Geometry check sheet. Reference: the model listing, model coordinates, mm. Face numbers are marked on the shaded views. A direction names the side the tool comes from. Coordinates: 2 decimals unless noted, no trailing zeros. Write each loop counter-clockwise with the first axis right and the second up, starting at its lowest first coordinate (ties: lowest second). Pieces come first, ordered by that corner, then holes. Notation, with made-up numbers: M 31.5,31.25 L 60.5,31.25 A18 cw 60.5,42.25 Z; hole C 28.25,-31.75 d9. An arc over 180 degrees is marked long. Put each result on its own line as item: value. Start each with the question number.
1) Cross-section at B-B on x = 0. Record the cut outline in (y, z).
2) Cross-section at C-C on y = 4. Count the separate pieces of the cut face and the enclosed holes in it, plus the area to 3 significant figures.
3) Set-up check for the marked faces 4, 5 and 6: record each of +Z, -Z, +X, -X, +Y, -Y from which the full face is reachable in a straight line by a thin tool's end or side.
4) Gauge pin test, flat ends, axial feed: pin 1 (1.6 mm diameter, centred on x = -7.5, z = 26.4, fed in from +Y); pin 2 (7 mm diameter, centred on x = 18, y = -4.5, fed in from -Z); pin 3 (7 mm diameter, centred on x = 16.5, y = -3, fed in from +Z). Record the tip position at first contact, or that the pin passes through.
5) Mould release check, pull along Z, two halves, no side actions. Record for the marked faces 1, 2 and 3: released by +Z, released by -Z, zero draft, split by the parting line, or undercut.
6) Cross-section at A-A on z = -5. Record the cut outline in (x, y), plus the area to 4 significant figures.
7) Scan lines: line 1 along X through (y, z) = (5, 29); line 2 along X through (y, z) = (-1.75, -5.5); line 3 along Z through (x, y) = (-22.5, -1.25). Record each from-to range of solid material in increasing order.
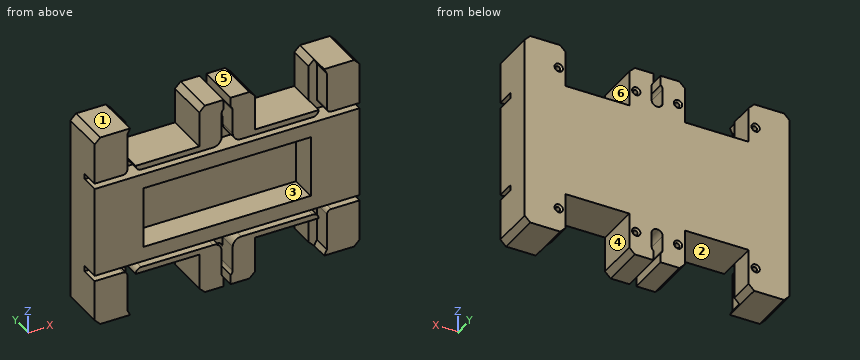
from build123d import *
from build123d.topology import SkipClean

# Parameters (mm, degrees)
SKETCH1_W            = 95
SKETCH1_H            = 70
BOSS_EXTRUDE1_DEPTH  = 7.85
CUT_EXTRUDE1_DEPTH   = 62.055220907
CHAMFER1_SIZE        = 2
CUT_EXTRUDE2_DEPTH   = 6.5
CUT_EXTRUDE3_DEPTH   = 60.715073474
MIRROR3_COPY_1_DEPTH = 6.5
SKETCH7_W            = 60
SKETCH7_H            = 22
CUT_EXTRUDE4_DEPTH   = 9.5


# Read off the part's stored shape, not the designer's step: CSK for M2 Flat Head Machine Screw1
with BuildPart() as part:
    # Sketch1 → Boss-Extrude1 (new, symmetric)
    with BuildSketch(Plane(origin=(0, 0, 0), x_dir=(1, 0, 0), z_dir=(0, 1, 0))):
        Rectangle(SKETCH1_W, SKETCH1_H)
    extrude(amount=BOSS_EXTRUDE1_DEPTH, both=True)

    # Sketch2 → Cut-Extrude1 (cut, through all)
    with BuildSketch(Plane(origin=(0, 7.85, 0), x_dir=(1, 0, 0), z_dir=(0, 1, 0))):
        Polygon((-32.8, -32.5), (-32.8, -20.3), (-10, -20.3), (-10, -32.5), (-10, -35), (-32.8, -35), align=None)
        Polygon((10, -32.5), (10, -20.3), (32.8, -20.3), (32.8, -32.5), (32.8, -35), (10, -35), align=None)
    cut_extrude1 = extrude(amount=-CUT_EXTRUDE1_DEPTH, mode=Mode.SUBTRACT)

    # CSK for M2 Flat Head Machine Screw1 outl → CSK for M2 Flat Head Machine Screw1 (revolve, cut)
    with BuildSketch(Plane(origin=(35.3, 0, 26.4), x_dir=(1, 0, 0), z_dir=(0, 0, 1))):
        Polygon((0, 7.85), (0, -0.672748739), (0.87, -0.15), (0.87, 7.22), (1.5, 7.85), align=None)
    csk_for_m2_flat_head_machine_screw1 = revolve(axis=Axis((35.3, 0, 26.4), (0, 1, 0)), mode=Mode.SUBTRACT)

    # CSK for M2 Flat Head Machine Screw1 2 ou → CSK for M2 Flat Head Machine Screw1 2 (revolve, cut)
    with BuildSketch(Plane(origin=(7.5, 0, 26.4), x_dir=(1, 0, 0), z_dir=(0, 0, 1))):
        Polygon((0, 7.85), (0, -0.672748739), (0.87, -0.15), (0.87, 7.22), (1.5, 7.85), align=None)
    csk_for_m2_flat_head_machine_screw1_2 = revolve(axis=Axis((7.5, 0, 26.4), (0, 1, 0)), mode=Mode.SUBTRACT)

    # CSK for M2 Flat Head Machine Screw1 3 ou → CSK for M2 Flat Head Machine Screw1 3 (revolve, cut)
    with BuildSketch(Plane(origin=(-7.5, 0, 26.4), x_dir=(1, 0, 0), z_dir=(0, 0, 1))):
        Polygon((0, 7.85), (0, -0.672748739), (0.87, -0.15), (0.87, 7.22), (1.5, 7.85), align=None)
    csk_for_m2_flat_head_machine_screw1_3 = revolve(axis=Axis((-7.5, 0, 26.4), (0, 1, 0)), mode=Mode.SUBTRACT)

    # CSK for M2 Flat Head Machine Screw1 4 ou → CSK for M2 Flat Head Machine Screw1 4 (revolve, cut)
    with BuildSketch(Plane(origin=(-35.3, 0, 26.4), x_dir=(1, 0, 0), z_dir=(0, 0, 1))):
        Polygon((0, 7.85), (0, -0.672748739), (0.87, -0.15), (0.87, 7.22), (1.5, 7.85), align=None)
    csk_for_m2_flat_head_machine_screw1_4 = revolve(axis=Axis((-35.3, 0, 26.4), (0, 1, 0)), mode=Mode.SUBTRACT)

    # Mirror1: Cut-Extrude1, CSK for M2 Flat Head Machine Screw1, CSK for M2 Flat Head Machine Screw1 2, CSK for M2 Flat Head Machine Screw1 3, CSK for M2 Flat Head Machine Screw1 4 across plane
    add(cut_extrude1.mirror(Plane.XY), mode=Mode.SUBTRACT)
    add(csk_for_m2_flat_head_machine_screw1.mirror(Plane.XY), mode=Mode.SUBTRACT)
    add(csk_for_m2_flat_head_machine_screw1_2.mirror(Plane.XY), mode=Mode.SUBTRACT)
    add(csk_for_m2_flat_head_machine_screw1_3.mirror(Plane.XY), mode=Mode.SUBTRACT)
    add(csk_for_m2_flat_head_machine_screw1_4.mirror(Plane.XY), mode=Mode.SUBTRACT)

    # Chamfer1
    chamfer1_edges = [part.edges().sort_by_distance(p)[0] for p in [
        (-32.8, 0, 35),
        (-10, 0, 35),
        (10, 0, 35),
        (32.8, 0, 35),
        (47.5, 0, 35),
        (-47.5, 0, 35),
        (-47.5, 0, -35),
        (47.5, 0, -35),
        (-32.8, 0, -35),
        (-10, 0, -35),
        (10, 0, -35),
        (32.8, 0, -35),
    ]]
    chamfer(chamfer1_edges, length=CHAMFER1_SIZE)

    # Sketch5 → Cut-Extrude2 (cut)
    with BuildSketch(Plane.XZ.offset(7.85)):
        with BuildLine():
            Line((47.5, 16.3), (-2, 16.3))
            Line((-2, 16.3), (-2, 30))
            ThreePointArc((-2, 30), (0, 32), (2, 30))
            Line((2, 30), (2, 21.3))
            ThreePointArc((2, 21.3), (2.878679656, 19.178679656), (5, 18.3))
            Line((5, 18.3), (30.8, 18.3))
            ThreePointArc((30.8, 18.3), (32.214213562, 18.885786438), (32.8, 20.3))
            Line((32.8, 20.3), (32.8, 33))
            Line((32.8, 33), (34.8, 35))
            Line((34.8, 35), (35.8, 33))
            Line((35.8, 33), (35.8, 19.8))
            ThreePointArc((35.8, 19.8), (36.239339828, 18.739339828), (37.3, 18.3))
            Line((37.3, 18.3), (47.5, 18.3))
            Line((47.5, 18.3), (47.5, 16.3))
        make_face()
    cut_extrude2 = extrude(amount=-CUT_EXTRUDE2_DEPTH, mode=Mode.SUBTRACT)

    # Sketch6 → Cut-Extrude3 (cut, symmetric)
    with SkipClean():  # the faces are left unmerged after this step: merging them gives an invalid solid
        with BuildSketch(Plane.XZ.offset(1.35)):
            with BuildLine():
                Line((2, 25), (2, 30))
                ThreePointArc((2, 30), (1.802775638, 30.866025404), (1.25, 31.5612495))
                Line((1.25, 31.5612495), (1.25, 35))
                Line((1.25, 35), (-1.25, 35))
                Line((-1.25, 35), (-1.25, 31.5612495))
                ThreePointArc((-1.25, 31.5612495), (-1.802775638, 30.866025404), (-2, 30))
                Line((-2, 30), (-2, 25))
                ThreePointArc((-2, 25), (0, 23), (2, 25))
            make_face()
        cut_extrude3 = extrude(amount=CUT_EXTRUDE3_DEPTH, both=True, mode=Mode.SUBTRACT)
    add(part.part.scale(1), mode=Mode.REPLACE)  # the faces are merged on a copy

    # Mirror2: Cut-Extrude2 across plane
    add(cut_extrude2.mirror(Plane(origin=(0, 0, 0), x_dir=(0, 0, 1), z_dir=(1, 0, 0))), mode=Mode.SUBTRACT)

    # Mirror3: Cut-Extrude2, Cut-Extrude3 across plane
    add(cut_extrude2.mirror(Plane.XY), mode=Mode.SUBTRACT)
    add(cut_extrude3.mirror(Plane.XY), mode=Mode.SUBTRACT)

    # Mirror3 copy 1 sketch → Mirror3 copy 1 (cut)
    with BuildSketch(Plane(origin=(0, -7.85, 0), x_dir=(-1, 0, 0), z_dir=(0, -1, 0))):
        with BuildLine():
            Line((47.5, 16.3), (-2, 16.3))
            Line((-2, 16.3), (-2, 30))
            ThreePointArc((-2, 30), (0, 32), (2, 30))
            Line((2, 30), (2, 21.3))
            ThreePointArc((2, 21.3), (2.878679656, 19.178679656), (5, 18.3))
            Line((5, 18.3), (30.8, 18.3))
            ThreePointArc((30.8, 18.3), (32.214213562, 18.885786438), (32.8, 20.3))
            Line((32.8, 20.3), (32.8, 33))
            Line((32.8, 33), (34.8, 35))
            Line((34.8, 35), (35.8, 33))
            Line((35.8, 33), (35.8, 19.8))
            ThreePointArc((35.8, 19.8), (36.239339828, 18.739339828), (37.3, 18.3))
            Line((37.3, 18.3), (47.5, 18.3))
            Line((47.5, 18.3), (47.5, 16.3))
        make_face()
    extrude(amount=-MIRROR3_COPY_1_DEPTH, mode=Mode.SUBTRACT)

    # Sketch7 → Cut-Extrude4 (cut)
    with BuildSketch(Plane.XZ.offset(7.85)):
        Rectangle(SKETCH7_W, SKETCH7_H)
    extrude(amount=-CUT_EXTRUDE4_DEPTH, mode=Mode.SUBTRACT)


solid = part.part
Answer key:
1. outline: M -7.85,-16.3 L -1.35,-16.3 L -1.35,-23 L 7.85,-23 L 7.85,23 L -1.35,23 L -1.35,16.3 L -7.85,16.3 L -7.85,11 L 1.65,11 L 1.65,-11 L -7.85,-11 Z
2. separate pieces: 1
2. enclosed holes: 8
2. area: 5,190 mm²
3. face 4: -Z, +Y, -Y
3. face 5: +Z, +X, -X, +Y, -Y
3. face 6: +Z, +Y, -Y
4. pin 1: stops at y = -0.19
4. pin 2: stops at z = -20.3
4. pin 3: stops at z = 20.3
5. face 1: released by +Z
5. face 2: released by -Z
5. face 3: undercut
6. outline: M -47.5,-7.85 L -30,-7.85 L -30,1.65 L 30,1.65 L 30,-7.85 L 47.5,-7.85 L 47.5,7.85 L -47.5,7.85 Z
6. area: 921.5 mm²
7. line 1: x = -47.5 to -32.8, -10 to -2, 2 to 10, 32.8 to 47.5
7. line 2: x = -47.5 to -30, 30 to 47.5
7. line 3: z = -20.3 to -11, 11 to 20.3
